For this review, take the finished solid that the model builds, in its own axes (mm). Face numbers are marked on the shaded views. A direction names the side the tool comes from. Coordinates: 2 decimals unless noted, no trailing zeros. Loops run counter-clockwise (first coordinate to the right, second up) from the corner with the lowest first, then second, coordinate; pieces in that order, holes last. Notation, with made-up numbers: M -25.5,19 L 17.5,19 A4 cw 17.5,26 Z; hole C -38.5,82 d6. An arc over 180 degrees is marked long. Write each question's results on one line, items separated by ' | '. Start each with the question number.
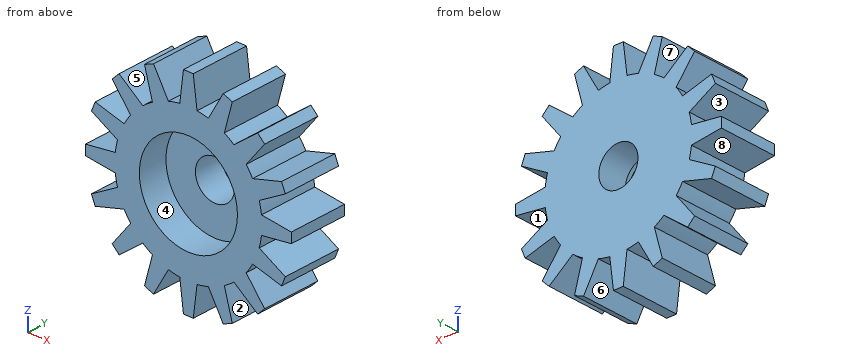
```python
from build123d import *

# Parameters (mm, degrees)
SKICA1_R                 = 3.75
P_IDAT_VYSUNUT_M1_DEPTH  = 3
P_IDAT_VYSUNUT_M2_DEPTH  = 3
KRUHOV_POLE1_COUNT       = 16
SKICA3_R                 = 1
ODEBRAT_VYSUNUT_M1_DEPTH = 5
SKICA4_R                 = 2.5
ODEBRAT_VYSUNUT_M2_DEPTH = 1.5


with BuildPart() as part:
    # Skica1 → Přidat vysunutím1 (new body)
    with BuildSketch(Plane(origin=(0, 0, 0), x_dir=(1, 0, 0), z_dir=(0, 1, 0))):
        Circle(SKICA1_R)
    extrude(amount=P_IDAT_VYSUNUT_M1_DEPTH)

    # Skica2 → Přidat vysunutím2 (add)
    with BuildSketch(Plane(origin=(0, 3, 0), x_dir=(1, 0, 0), z_dir=(0, 1, 0))):
        with BuildLine():
            Line((0, 5.244044241), (0.25, 5.244044241))
            Line((0.25, 5.244044241), (0.439992833, 3.724098053))
            ThreePointArc((0.439992833, 3.724098053), (0, 3.75), (-0.439992833, 3.724098053))
            Line((-0.439992833, 3.724098053), (-0.25, 5.244044241))
            Line((-0.25, 5.244044241), (0, 5.244044241))
        make_face()
    p_idat_vysunut_m2 = extrude(amount=-P_IDAT_VYSUNUT_M2_DEPTH)

    # Kruhové pole1: Přidat vysunutím2 ×16 about axis
    kruhov_pole1_axis = Axis((0, 0, 0), (0, 1, 0))
    for i in range(1, KRUHOV_POLE1_COUNT):
        add(p_idat_vysunut_m2.rotate(kruhov_pole1_axis, i * 360 / KRUHOV_POLE1_COUNT))

    # Skica3 → Odebrat vysunutím1 (cut)
    with BuildSketch(Plane.XZ):
        Circle(SKICA3_R)
    extrude(amount=-ODEBRAT_VYSUNUT_M1_DEPTH, mode=Mode.SUBTRACT)

    # Skica4 → Odebrat vysunutím2 (cut)
    with BuildSketch(Plane.XZ):
        Circle(SKICA4_R)
    extrude(amount=-ODEBRAT_VYSUNUT_M2_DEPTH, mode=Mode.SUBTRACT)


solid = part.part
```
Q1. Take a section at B-B, the plane x = 0. Give the boundary of the cut face in (y, z), then the cut area to 3 significant figures.
Q2. The part is to be moulded in two halves that separate along Z. For the marked faces 5, 6, 7 and 8, say which applies: pulls with the +Z half, pulls with the -Z half, needs draft (parallel to the pull), parting line crosses it, or undercut.
Q3. To check wall thickness, follow line 1 along Z through (x, y) = (0, 1); line 2 along Z through (x, y) = (0, 2.6); line 3 along Z through (x, y) = (3.5, 2.85). State the ranges of each line that lie inside material, in increasing order.
Q4. Take a section at A-A, the plane z = 0. Give the boundary of the cut face in (x, y), then the cut area to 3 significant figures.
Q5. Take a section at C-C, the plane z = 1.5. Give the boundary of the cut face in (x, y).
Q6. For the marked faces 1, 2, 3 and 4, list the 3-axis set-ups (+Z, -Z, +X, -X, +Y, -Y) from which the entire face can be reached by the end or side of a thin tool; tool diameter is ignored.
Q7. Take a section at D-D, the plane x = 1.25. Give the boundary of the cut face in (y, z), then the cut area to 3 significant figures.
Q8. Insertion check: P1, Ø1.5, axis at y = 1, z = -0.5, coming from the +X side. The pin has a flat end and moves straight along its axis. Give the tip position at first contact, or say it passes through.
Results:
1) outline: M 0,-5.24 L 3,-5.24 L 3,-1 L 1.5,-1 L 1.5,-2.5 L 0,-2.5 Z; M 0,2.5 L 1.5,2.5 L 1.5,1 L 3,1 L 3,5.24 L 0,5.24 Z | area: 21.0 mm^2
2) face 5: pulls with the +Z half | face 6: pulls with the -Z half | face 7: undercut | face 8: undercut
3) line 1: -5.24 to -2.5, 2.5 to 5.24 | line 2: -5.24 to -1, 1 to 5.24 | line 3: -3.86 to -3.04, -1.89 to 1.89, 3.04 to 3.86
4) outline: M -5.24,0 L -2.5,0 L -2.5,1.5 L -1,1.5 L -1,3 L -5.24,3 Z; M 1,1.5 L 2.5,1.5 L 2.5,0 L 5.24,0 L 5.24,3 L 1,3 Z | area: 21.0 mm^2
5) outline: M -4.46,0 L -2,0 L -2,1.5 L 2,1.5 L 2,0 L 4.46,0 L 4.46,3 L -4.46,3 Z
6) face 1: +X, +Y, -Y | face 2: +Y, -Y | face 3: -X, +Y, -Y | face 4: -Y
7) outline: M 0,-4.02 L 3,-4.02 L 3,4.02 L 0,4.02 L 0,2.17 L 1.5,2.17 L 1.5,-2.17 L 0,-2.17 Z | area: 17.6 mm^2
8) P1: x = 5.24
